Source: CAD feature listing. Evaluate the final solid. Frame: model axes, mm. A direction names the side the tool comes from. Give positions to 0.01 mm unless a question says otherwise; leave off trailing zeros. Order: outer loops, then holes, each group sorted by start corner. A loop starts at its lowest first (then second) coordinate and runs counter-clockwise, first axis right, second up. Notation, with made-up numbers: M 86.25,8.5 L 144.25,8.5 A8 cw 144.25,22.5 Z; hole C 39.25,73.5 d8. An arc over 180 degrees is marked long. Use CSV: the item, a comma, the result in double quotes. Start each with the question number.
Item 1: First-contact query: pin 1 (2 mm diameter, centred on x = 11.5, z = -12.5, fed in from +Y); pin 2 (2.5 mm diameter, centred on x = 7, z = -9, fed in from +Y). Flat tips, straight axial feed; report the tip coordinate or a pass-through.
Item 2: Section query C-C on x = 46.5. Return loops of the section in (y, z).
Item 3: Access query for faces 1 (the face through (52, 32, -70)), 2 (the face through (2, 49, -35)). Directions: +Z, -Z, +X, -X, +Y, -Y. A direction counts if a zero-diameter tool reaches every point of the face in a straight line with its end or side. Return the directions, or none.
Item 4: Pull-direction query (Z, two-part tool) for faces 3 (the face through (36, 65, -1)), 4 (the face through (51, 32, 0)), 5 (the face through (100, 16, -35)); classes: +Z half, -Z half, draft (parallel to the pull), parting line (faces both ways), or undercut.
Item 5: Section query D-D on z = -48.5. Return loops of the section in (x, y), and give its area (4 significant figures).
Item 6: Ray query, probe 1 along X at (y, z) = (44.5, -10); probe 2 along Z at (x, y) = (97.5, 12); probe 3 along Z at (x, y) = (11, 29). Return the intervals inside material, ascending. Write a range as from..to.
Item 7: Section query A-A on y = 3.5. Return loops of the section in (x, z), and give its area (3 significant figures).
Item 8: Section query B-B on z = -62. Return loops of the section in (x, y).
from build123d import *

# Parameters (mm, degrees)
SKETCH1_W            = 97
SKETCH1_H            = 64
SKETCH1_R            = 4
SKETCH1_R_2          = 2
BOSS_EXTRUDE4_DEPTH  = 2.5
BOSS_EXTRUDE5_START  = 65
BOSS_EXTRUDE5_DEPTH  = 65
BOSS_EXTRUDE6_START  = 32
SKETCH1_9_W          = 97
SKETCH1_9_H          = 64
SKETCH1_9_R          = 4
SKETCH1_9_R_2        = 2
BOSS_EXTRUDE6_DEPTH  = 32
SKETCH3_R            = 2
BOSS_EXTRUDE7_DEPTH  = 5
SKETCH6_R            = 2
BOSS_EXTRUDE8_DEPTH  = 5
SKETCH5_R            = 2
BOSS_EXTRUDE9_DEPTH  = 5
SKETCH4_R            = 2
BOSS_EXTRUDE10_DEPTH = 5


with BuildPart() as part:
    # Sketch1 → Boss-Extrude4 (new body)
    # profile 1 of 11: a face of its own
    with BuildSketch(Plane(origin=(0, 0, 0), x_dir=(1, 0, 0), z_dir=(0, 1, 0))):
        with BuildLine():
            Line((103, 3), (103, 67))
            ThreePointArc((103, 67), (102.121320344, 69.121320344), (100, 70))
            Line((100, 70), (3, 70))
            ThreePointArc((3, 70), (0.878679656, 69.121320344), (0, 67))
            Line((0, 67), (0, 3))
            ThreePointArc((0, 3), (0.878679656, 0.878679656), (3, 0))
            Line((3, 0), (100, 0))
            ThreePointArc((100, 0), (102.121320344, 0.878679656), (103, 3))
        make_face()
        with BuildLine():
            Line((3, 2), (100, 2))
            ThreePointArc((100, 2), (100.707106781, 2.292893219), (101, 3))
            Line((101, 3), (101, 67))
            ThreePointArc((101, 67), (100.707106781, 67.707106781), (100, 68))
            Line((100, 68), (3, 68))
            ThreePointArc((3, 68), (2.292893219, 67.707106781), (2, 67))
            Line((2, 67), (2, 3))
            ThreePointArc((2, 3), (2.292893219, 2.292893219), (3, 2))
        make_face(mode=Mode.SUBTRACT)
    # profile 2 of 11: a face of its own
    with BuildSketch(Plane(origin=(0, 0, 0), x_dir=(1, 0, 0), z_dir=(0, 1, 0))):
        with BuildLine():
            ThreePointArc((3, 2), (2.292893219, 2.292893219), (2, 3))
            Line((2, 3), (2, 67))
            ThreePointArc((2, 67), (2.292893219, 67.707106781), (3, 68))
            Line((3, 68), (100, 68))
            ThreePointArc((100, 68), (100.707106781, 67.707106781), (101, 67))
            Line((101, 67), (101, 3))
            ThreePointArc((101, 3), (100.707106781, 2.292893219), (100, 2))
            Line((100, 2), (3, 2))
        make_face()
        with Locations((51.5, 35)):
            Rectangle(SKETCH1_W, SKETCH1_H, mode=Mode.SUBTRACT)
    # profile 3 of 11: a face of its own
    with BuildSketch(Plane(origin=(0, 0, 0), x_dir=(1, 0, 0), z_dir=(0, 1, 0))):
        with Locations((51.5, 35)):
            Rectangle(SKETCH1_W, SKETCH1_H)
        with Locations((95, 62)):
            Circle(SKETCH1_R, mode=Mode.SUBTRACT)
        with Locations((95, 8)):
            Circle(SKETCH1_R, mode=Mode.SUBTRACT)
        with Locations((8, 62)):
            Circle(SKETCH1_R, mode=Mode.SUBTRACT)
        with Locations((8, 8)):
            Circle(SKETCH1_R, mode=Mode.SUBTRACT)
    # profile 4 of 11: a face of its own
    with BuildSketch(Plane(origin=(0, 0, 0), x_dir=(1, 0, 0), z_dir=(0, 1, 0))):
        with Locations((8, 8)):
            Circle(SKETCH1_R)
        with Locations((8, 8)):
            Circle(SKETCH1_R_2, mode=Mode.SUBTRACT)
    # profile 5 of 11: a face of its own
    with BuildSketch(Plane(origin=(0, 0, 0), x_dir=(1, 0, 0), z_dir=(0, 1, 0))):
        with Locations((8, 8)):
            Circle(SKETCH1_R_2)
    # profile 6 of 11: a face of its own
    with BuildSketch(Plane(origin=(0, 0, 0), x_dir=(1, 0, 0), z_dir=(0, 1, 0))):
        with Locations((95, 8)):
            Circle(SKETCH1_R)
        with Locations((95, 8)):
            Circle(SKETCH1_R_2, mode=Mode.SUBTRACT)
    # profile 7 of 11: a face of its own
    with BuildSketch(Plane(origin=(0, 0, 0), x_dir=(1, 0, 0), z_dir=(0, 1, 0))):
        with Locations((95, 8)):
            Circle(SKETCH1_R_2)
    # profile 8 of 11: a face of its own
    with BuildSketch(Plane(origin=(0, 0, 0), x_dir=(1, 0, 0), z_dir=(0, 1, 0))):
        with Locations((95, 62)):
            Circle(SKETCH1_R)
        with Locations((95, 62)):
            Circle(SKETCH1_R_2, mode=Mode.SUBTRACT)
    # profile 9 of 11: a face of its own
    with BuildSketch(Plane(origin=(0, 0, 0), x_dir=(1, 0, 0), z_dir=(0, 1, 0))):
        with Locations((95, 62)):
            Circle(SKETCH1_R_2)
    # profile 10 of 11: a face of its own
    with BuildSketch(Plane(origin=(0, 0, 0), x_dir=(1, 0, 0), z_dir=(0, 1, 0))):
        with Locations((8, 62)):
            Circle(SKETCH1_R)
        with Locations((8, 62)):
            Circle(SKETCH1_R_2, mode=Mode.SUBTRACT)
    # profile 11 of 11: a face of its own
    with BuildSketch(Plane(origin=(0, 0, 0), x_dir=(1, 0, 0), z_dir=(0, 1, 0))):
        with Locations((8, 62)):
            Circle(SKETCH1_R_2)
    extrude(amount=-BOSS_EXTRUDE4_DEPTH)

    # Sketch1_8 → Boss-Extrude5 (add)
    with BuildSketch(Plane(origin=(0, 0, 0), x_dir=(1, 0, 0), z_dir=(0, 1, 0)).offset(BOSS_EXTRUDE5_START)):
        with BuildLine():
            Line((103, 3), (103, 67))
            ThreePointArc((103, 67), (102.121320344, 69.121320344), (100, 70))
            Line((100, 70), (3, 70))
            ThreePointArc((3, 70), (0.878679656, 69.121320344), (0, 67))
            Line((0, 67), (0, 3))
            ThreePointArc((0, 3), (0.878679656, 0.878679656), (3, 0))
            Line((3, 0), (100, 0))
            ThreePointArc((100, 0), (102.121320344, 0.878679656), (103, 3))
        make_face()
        with BuildLine():
            Line((3, 2), (100, 2))
            ThreePointArc((100, 2), (100.707106781, 2.292893219), (101, 3))
            Line((101, 3), (101, 67))
            ThreePointArc((101, 67), (100.707106781, 67.707106781), (100, 68))
            Line((100, 68), (3, 68))
            ThreePointArc((3, 68), (2.292893219, 67.707106781), (2, 67))
            Line((2, 67), (2, 3))
            ThreePointArc((2, 3), (2.292893219, 2.292893219), (3, 2))
        make_face(mode=Mode.SUBTRACT)
    extrude(amount=-BOSS_EXTRUDE5_DEPTH)

    # Sketch1_9 → Boss-Extrude6 (add)
    # profile 1 of 9: a face of its own
    with BuildSketch(Plane(origin=(0, 0, 0), x_dir=(1, 0, 0), z_dir=(0, 1, 0)).offset(BOSS_EXTRUDE6_START)):
        with BuildLine():
            ThreePointArc((3, 2), (2.292893219, 2.292893219), (2, 3))
            Line((2, 3), (2, 67))
            ThreePointArc((2, 67), (2.292893219, 67.707106781), (3, 68))
            Line((3, 68), (100, 68))
            ThreePointArc((100, 68), (100.707106781, 67.707106781), (101, 67))
            Line((101, 67), (101, 3))
            ThreePointArc((101, 3), (100.707106781, 2.292893219), (100, 2))
            Line((100, 2), (3, 2))
        make_face()
        with Locations((51.5, 35)):
            Rectangle(SKETCH1_9_W, SKETCH1_9_H, mode=Mode.SUBTRACT)
    # profile 2 of 9: a face of its own
    with BuildSketch(Plane(origin=(0, 0, 0), x_dir=(1, 0, 0), z_dir=(0, 1, 0)).offset(BOSS_EXTRUDE6_START)):
        with Locations(Location((8, 62, 0), (0, 0, 270))):
            Circle(SKETCH1_9_R)
        with Locations((8, 62)):
            Circle(SKETCH1_9_R_2, mode=Mode.SUBTRACT)
    # profile 3 of 9: a face of its own
    with BuildSketch(Plane(origin=(0, 0, 0), x_dir=(1, 0, 0), z_dir=(0, 1, 0)).offset(BOSS_EXTRUDE6_START)):
        with Locations((8, 62)):
            Circle(SKETCH1_9_R_2)
    # profile 4 of 9: a face of its own
    with BuildSketch(Plane(origin=(0, 0, 0), x_dir=(1, 0, 0), z_dir=(0, 1, 0)).offset(BOSS_EXTRUDE6_START)):
        with Locations(Location((95, 62, 0), (0, 0, 270))):
            Circle(SKETCH1_9_R)
        with Locations((95, 62)):
            Circle(SKETCH1_9_R_2, mode=Mode.SUBTRACT)
    # profile 5 of 9: a face of its own
    with BuildSketch(Plane(origin=(0, 0, 0), x_dir=(1, 0, 0), z_dir=(0, 1, 0)).offset(BOSS_EXTRUDE6_START)):
        with Locations((95, 62)):
            Circle(SKETCH1_9_R_2)
    # profile 6 of 9: a face of its own
    with BuildSketch(Plane(origin=(0, 0, 0), x_dir=(1, 0, 0), z_dir=(0, 1, 0)).offset(BOSS_EXTRUDE6_START)):
        with Locations(Location((95, 8, 0), (0, 0, 270))):
            Circle(SKETCH1_9_R)
        with Locations((95, 8)):
            Circle(SKETCH1_9_R_2, mode=Mode.SUBTRACT)
    # profile 7 of 9: a face of its own
    with BuildSketch(Plane(origin=(0, 0, 0), x_dir=(1, 0, 0), z_dir=(0, 1, 0)).offset(BOSS_EXTRUDE6_START)):
        with Locations((95, 8)):
            Circle(SKETCH1_9_R_2)
    # profile 8 of 9: a face of its own
    with BuildSketch(Plane(origin=(0, 0, 0), x_dir=(1, 0, 0), z_dir=(0, 1, 0)).offset(BOSS_EXTRUDE6_START)):
        with Locations(Location((8, 8, 0), (0, 0, 270))):
            Circle(SKETCH1_9_R)
        with Locations((8, 8)):
            Circle(SKETCH1_9_R_2, mode=Mode.SUBTRACT)
    # profile 9 of 9: a face of its own
    with BuildSketch(Plane(origin=(0, 0, 0), x_dir=(1, 0, 0), z_dir=(0, 1, 0)).offset(BOSS_EXTRUDE6_START)):
        with Locations((8, 8)):
            Circle(SKETCH1_9_R_2)
    extrude(amount=-BOSS_EXTRUDE6_DEPTH)

    # Sketch3 → Boss-Extrude7 (add)
    with BuildSketch(Plane(origin=(0, 32, 0), x_dir=(1, 0, 0), z_dir=(0, 1, 0))):
        with Locations(Location((8, 62, 0), (0, 0, 270))):
            Circle(SKETCH3_R)
    extrude(amount=BOSS_EXTRUDE7_DEPTH)

    # Sketch6 → Boss-Extrude8 (add)
    with BuildSketch(Plane(origin=(0, 32, 0), x_dir=(1, 0, 0), z_dir=(0, 1, 0))):
        with Locations(Location((95, 62, 0), (0, 0, 270))):
            Circle(SKETCH6_R)
    extrude(amount=BOSS_EXTRUDE8_DEPTH)

    # Sketch5 → Boss-Extrude9 (add)
    with BuildSketch(Plane(origin=(0, 32, 0), x_dir=(1, 0, 0), z_dir=(0, 1, 0))):
        with Locations(Location((95, 8, 0), (0, 0, 270))):
            Circle(SKETCH5_R)
    extrude(amount=BOSS_EXTRUDE9_DEPTH)

    # Sketch4 → Boss-Extrude10 (add)
    with BuildSketch(Plane(origin=(0, 32, 0), x_dir=(1, 0, 0), z_dir=(0, 1, 0))):
        with Locations(Location((8, 8, 0), (0, 0, 270))):
            Circle(SKETCH4_R)
    extrude(amount=BOSS_EXTRUDE10_DEPTH)


solid = part.part
Verdict:
1,pin 1,"y = 0"
1,pin 2,"y = 37"
2,outline,"M -2.5,-70 L 65,-70 L 65,-68 L 32,-68 L 32,-67 L 0,-67 L 0,-3 L 32,-3 L 32,-2 L 65,-2 L 65,0 L -2.5,0 Z"
3,face 1,"-Z, +X, -X, +Y, -Y"
3,face 2,"+Y"
4,face 3,"draft"
4,face 4,"+Z half"
4,face 5,"undercut"
5,outline,"M 0,-2.5 L 103,-2.5 L 103,65 L 101,65 L 101,32 L 100,32 L 100,0 L 3,0 L 3,32 L 2,32 L 2,65 L 0,65 Z"
5,area,"581.5 mm2"
6,probe 1,"0..2, 101..103"
6,probe 2,"-70..-67, -65.12..-58.88, -11.12..-4.88, -3..0"
6,probe 3,"-70..-67, -64.65..-59.35, -10.65..-5.35, -3..0"
7,outline,"M 0,-67 A3 ccw 3,-70 L 100,-70 A3 ccw 103,-67 L 103,-3 A3 ccw 100,0 L 3,0 A3 ccw 0,-3 Z; C 8,-62 d8; C 8,-8 d8; C 95,-62 d8; C 95,-8 d8; hole M 3,-67 L 100,-67 L 100,-3 L 3,-3 Z"
7,area,"1,200 mm2"
8,outline,"M 0,-2.5 L 103,-2.5 L 103,65 L 101,65 L 101,32 L 100,32 L 100,0 L 99,0 L 99,32 L 97,32 L 97,37 L 93,37 L 93,32 L 91,32 L 91,0 L 12,0 L 12,32 L 10,32 L 10,37 L 6,37 L 6,32 L 4,32 L 4,0 L 3,0 L 3,32 L 2,32 L 2,65 L 0,65 Z"
